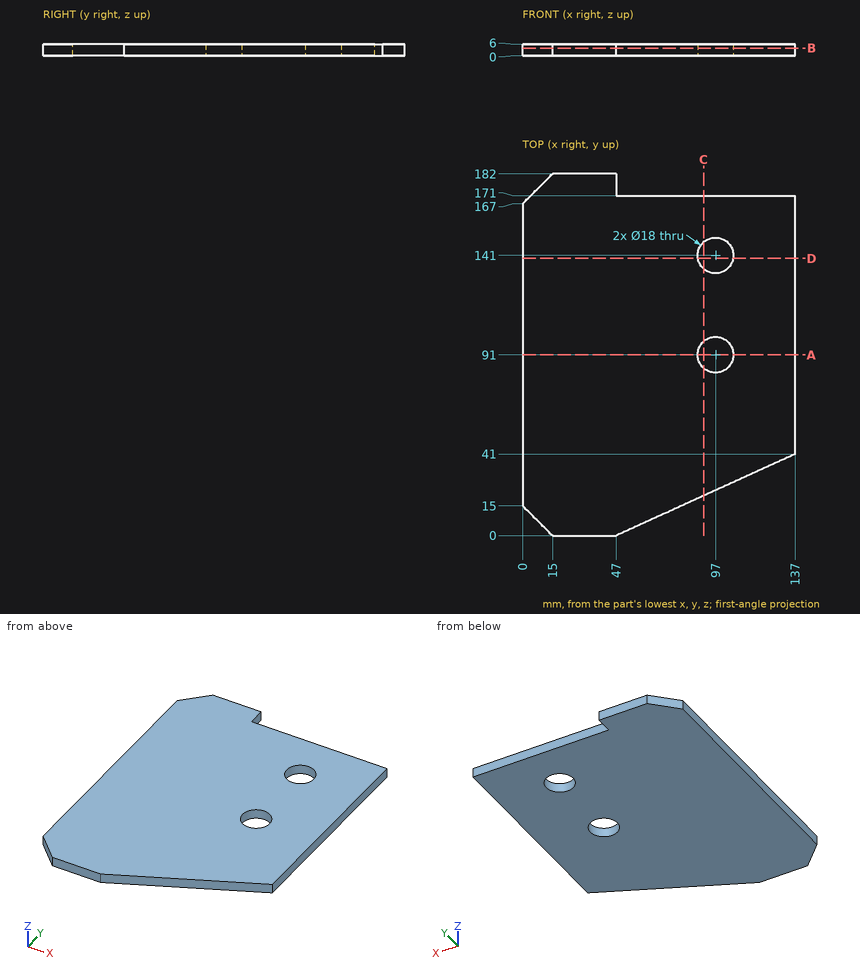
Can you work these out from the drawing? Everything is in mm from the part's minimum corner. Round coordinates to 2 decimals unless told otherwise and drop trailing zeros. Loops run counter-clockwise (first coordinate to the right, second up) from the corner with the lowest first, then second, coordinate; pieces in that order, holes last. Notation, with made-up numbers: (-34, 33.5) - (-8, 33.5) arc R20 cw to (-8, 49.5) - close; hole circle Ø7 at (69.25, -2). An arc over 180 degrees is marked (long way). Write item = value, one per line. Start each with the question number.
(1) If we section it at A-A (y = 91): Please give me the cut outline in (x, z), and give its area (3 significant figures).
(2) For P1, Ø1.5, axis at x = 116, z = 1, coming from the +Y side, with a flat end and sliding along its axis, tell me the tip position at first contact or that it passes through.
(3) If we section it at C-C (x = 91): Please give me the cut outline in (y, z), and give its area (3 significant figures).
(4) If I drill on probe 1 along X at (y, z) = (91, 3.75); probe 2 along Y at (x, z) = (97, 1.9); probe 3 along X at (y, z) = (93.5, 3.4), over which ranges is the centre line in solid material (lowest first)? Write a range as [from, to].
(5) If we section it at D-D (y = 139.5): Please give me the cut outline in (x, z), and give its area (3 significant figures).
(6) If we section it at B-B (z = 3.9): Please give me the cut outline in (x, y).
Ans:
q1.outline = (0, 0) - (88, 0) - (88, 6) - (0, 6) - close; (106, 0) - (137, 0) - (137, 6) - (106, 6) - close
q1.area = 714 mm²
q2.P1 = 171
q3.outline = (20.04, 0) - (84.29, 0) - (84.29, 6) - (20.04, 6) - close; (97.71, 0) - (134.29, 0) - (134.29, 6) - (97.71, 6) - close; (147.71, 0) - (171, 0) - (171, 6) - (147.71, 6) - close
q3.area = 745 mm²
q4.probe_1 = [0, 88], [106, 137]
q4.probe_2 = [22.78, 82], [100, 132], [150, 171]
q4.probe_3 = [0, 88.35], [105.65, 137]
q5.outline = (0, 0) - (88.13, 0) - (88.13, 6) - (0, 6) - close; (105.87, 0) - (137, 0) - (137, 6) - (105.87, 6) - close
q5.area = 716 mm²
q6.outline = (0, 15) - (15, 0) - (47, 0) - (137, 41) - (137, 171) - (47, 171) - (47, 182) - (15, 182) - (0, 167) - close; hole circle Ø18 at (97, 91); hole circle Ø18 at (97, 141)
